Job drawing, mm, ordinate dimensions from the low corner. One solid piece. Round coordinates to 2 decimals unless told otherwise and drop trailing zeros. Write each question's results on one line, items separated by ' | '. Start each with the question number.
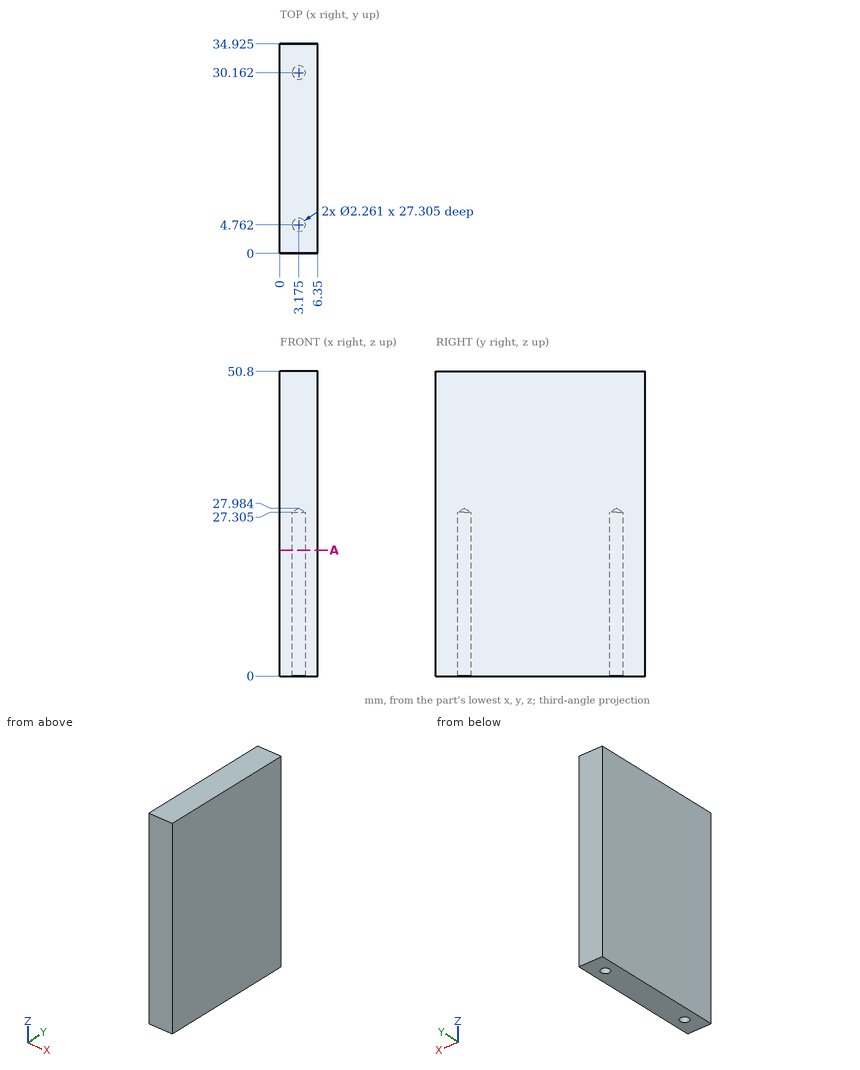
1) Wall check: line 1 along Y through (x, z) = (3.25, 8.5) (1 decimal); line 2 along Y through (x, z) = (3.75, 17) (1 decimal). Give the ranges that are in metal, low to high. Write a range as from..to.
2) Drop a flat-ended pin along its axis: pin 1 Ø2 at (x, y) = (3.18, 4.76) entering from -Z. Give the stop position or say it passes through.
3) Saw through at A-A, the plane z = 21. State how many separate pieces and enclosed holes the cut face has, plus the area to 3 significant figures.
Filled sheet:
1) line 1: y = 0..3.6, 5.9..29, 31.3..34.9 | line 2: y = 0..3.8, 5.7..29.2, 31.1..34.9
2) pin 1: stops at z = 27.38
3) separate pieces: 1 | enclosed holes: 2 | area: 214 mm^2
